```python
from build123d import *

# Parameters (mm, degrees)
EXTRUDE_1_DEPTH     = 62
SKETCH_2_W          = 31
SKETCH_2_H          = 23
CUT_EXTRUDE_1_DEPTH = 70
SKETCH_3_R          = 7
CUT_EXTRUDE_2_DEPTH = 62


with BuildPart() as part:
    # 스케치1 → 보스-돌출1 (new body)
    with BuildSketch(Plane.XY):
        Polygon((0, 0), (95, 0), (41, 46), (0, 46), align=None)
    extrude(amount=-EXTRUDE_1_DEPTH)

    # 스케치2 → 컷-돌출1 (cut)
    with BuildSketch(Plane.ZY):
        with Locations((-15.5, 34.5)):
            Rectangle(SKETCH_2_W, SKETCH_2_H)
    extrude(amount=-CUT_EXTRUDE_1_DEPTH, mode=Mode.SUBTRACT)

    # 스케치3 → 컷-돌출2 (cut)
    with BuildSketch(Plane(origin=(0, 23, 0), x_dir=(1, 0, 0), z_dir=(0, 1, 0))):
        with Locations(Location((21, 15, 0), (0, 0, 270))):
            Circle(SKETCH_3_R)
        with Locations(Location((47, 15, 0), (0, 0, 270))):
            Circle(SKETCH_3_R)
    extrude(amount=-CUT_EXTRUDE_2_DEPTH, mode=Mode.SUBTRACT)


solid = part.part
```
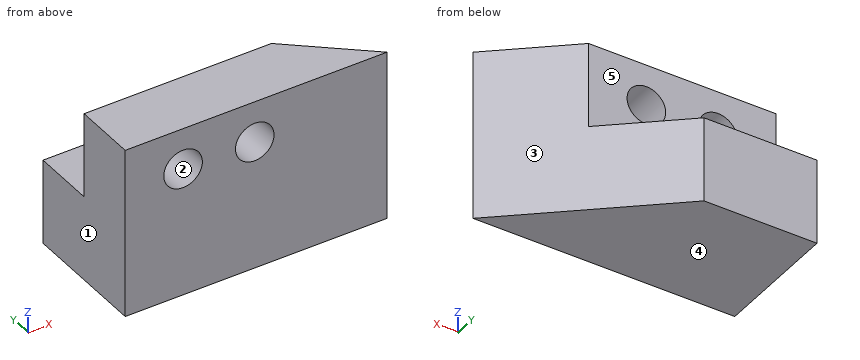
For this review, take the finished solid that the model builds, in its own axes (mm). Face numbers are marked on the shaded views. A direction names the side the tool comes from. Coordinates: 2 decimals unless noted, no trailing zeros. Order: outer loops, then holes, each group sorted by start corner. A loop starts at its lowest first (then second) coordinate and runs counter-clockwise, first axis right, second up. Notation, with made-up numbers: (81.25, -5.5) - (86.25, -5.5) arc R16 ccw to (86.25, 8.5) - close; hole circle Ø8 at (82, 11). An arc over 180 degrees is marked (long way). Answer as a JSON object with one key per item and string values. Group by question number.
1. We need section B-B on x = 21. State the section outline as (y, z) points, then the cut area to 3 significant figures.
2. Clearance check with flat-ended pins moving along their axes: P1, Ø1.5, axis at x = 67, z = -38.5, coming from the +Y side; P2, Ø8, axis at x = 43.5, y = 35, coming from the +Z side; P3, Ø2, axis at x = 57, z = -7.5, coming from the +Y side. State where each tip first meets the part, or that it passes through.
3. The part is to be moulded in two halves that separate along X. For the marked faces 1, 2 and 3, say which applies: pulls with the +X half, pulls with the -X half, needs draft (parallel to the pull), parting line crosses it, or undercut.
4. For the marked faces 4 and 5, list the 3-axis set-ups (+Z, -Z, +X, -X, +Y, -Y) from which the entire face can be reached by the end or side of a thin tool; tool diameter is ignored.
5. For probe 1 along X at (y, z) = (7.25, -15); probe 2 along X at (y, z) = (17, -15); probe 3 along Z at (x, y) = (53, 4), list the stretches that pass through material, from the lowest coordinate up.
6. We need section A-A on z = -15. State the section outline as (x, y) points, then the cut area to 3 significant figures.
7. We need section D-D on z = -45. State the section outline as (x, y) points.
8. We need section C-C on y = 13. State the section outline as (x, z) points, then the cut area to 3 significant figures.
Final values:
{
 "1": {"outline": "(0, -62) - (46, -62) - (46, -31) - (23, -31) - (23, -22) - (0, -22) - close; (0, -8) - (23, -8) - (23, 0) - (0, 0) - close", "area": "1,820 mm²"},
 "2": {"P1": "y = 24.49", "P2": "z = -31", "P3": "y = 23"},
 "3": {"face 1": "pulls with the -X half", "face 2": "undercut", "face 3": "pulls with the +X half"},
 "4": {"face 4": "-Z, +X, -X, +Y, -Y", "face 5": "+Z, +X, -X, +Y"},
 "5": {"probe 1": "0 to 14, 28 to 40, 54 to 86.49", "probe 2": "0 to 14, 28 to 40, 54 to 75.04", "probe 3": "-62 to -18.61, -11.39 to 0"},
 "6": {"outline": "(0, 0) - (14, 0) - (14, 23) - (0, 23) - close; (28, 0) - (40, 0) - (40, 23) - (28, 23) - close; (54, 0) - (95, 0) - (68, 23) - (54, 23) - close", "area": "1,230 mm²"},
 "7": {"outline": "(0, 0) - (95, 0) - (41, 46) - (0, 46) - close"},
 "8": {"outline": "(0, -62) - (79.74, -62) - (79.74, 0) - (0, 0) - close; hole circle Ø14 at (21, -15); hole circle Ø14 at (47, -15)", "area": "4,640 mm²"}
}
